Build history of the part. All positions in model axes, mm. Give positions to 0.01 mm unless a question says otherwise; leave off trailing zeros. Loops run counter-clockwise (first coordinate to the right, second up) from the corner with the lowest first, then second, coordinate; pieces in that order, holes last. Notation, with made-up numbers: M -11,33.25 L 1,33.25 A18 cw 1,67.25 Z; hole C 24,19 d8. An arc over 180 degrees is marked long. Answer in a Markdown table with one row per item. Add a question column.
```python
from build123d import *

# Parameters (mm, degrees)
SKETCH1_R           = 7.94
BOSS_EXTRUDE1_DEPTH = 100
SKETCH2_W           = 10.691765032
SKETCH2_H           = 3.27703882
SKETCH2_W_2         = 8.911923052
CUT_EXTRUDE1_DEPTH  = 101
FILLET1_R           = 1


with BuildPart() as part:
    # Sketch1 → Boss-Extrude1 (new body)
    with BuildSketch(Plane(origin=(0, 0, 0), x_dir=(0, 0, -1), z_dir=(1, 0, 0))):
        Circle(SKETCH1_R)
    extrude(amount=BOSS_EXTRUDE1_DEPTH)

    # Sketch2 → Cut-Extrude1 (cut, through all)
    with BuildSketch(Plane(origin=(100, 0, 0), x_dir=(0, 0, -1), z_dir=(1, 0, 0))):
        with Locations((-5.345882516, 7.57851941)):
            Rectangle(SKETCH2_W, SKETCH2_H)
        with Locations((4.455961526, 7.57851941)):
            Rectangle(SKETCH2_W_2, SKETCH2_H)
    extrude(amount=-CUT_EXTRUDE1_DEPTH, mode=Mode.SUBTRACT)

    # Fillet1
    fillet1_edges = [part.edges().sort_by_distance(p)[0] for p in [
        (50, 5.94, -5.268775949),
        (50, 5.94, 5.268775949),
    ]]
    fillet(fillet1_edges, radius=FILLET1_R)


solid = part.part
```
(1) Slice it at B-B, the plane y = -4.75. Give the cut face in (x, z), then the cut area to 3 significant figures.
(2) Pin check, flat tip, straight feed: pin 1 (2 mm diameter, centred on x = 23.5, y = -3, fed in from -Z). Stop position of the tip, or through.
(3) Slice it at A-A, the plane x = 58.5. Give the cut face in (y, z), then the cut area to 3 significant figures.
(4) Wall check: line 1 (Z direction, x = 6, y = 5.5); line 2 (Z direction, x = 71, y = -0.5); line 3 (Y direction, x = 58, z = 0.25). Give the ranges that are in metal, low to high.
Solution:
| question | item | result |
|---|---|---|
| 1 | outline | M 0,-6.36 L 100,-6.36 L 100,6.36 L 0,6.36 Z |
| 1 | area | 1,270 mm^2 |
| 2 | pin 1 | z = -7.68 |
| 3 | outline | M 5.65,-5.58 A1 ccw 5.94,-4.87 L 5.94,4.87 A1 ccw 5.65,5.58 A7.94 ccw long Z |
| 3 | area | 184 mm^2 |
| 4 | line 1 | -5.73 to 5.73 |
| 4 | line 2 | -7.92 to 7.92 |
| 4 | line 3 | -7.94 to 5.94 |
